The model under review builds one solid part; all positions refer to its coordinate system, in mm. Face numbers are marked on the shaded views. A direction names the side the tool comes from. Round coordinates to 2 decimals unless told otherwise and drop trailing zeros. Write each loop counter-clockwise with the first axis right and the second up, starting at its lowest first coordinate (ties: lowest second). Pieces come first, ordered by that corner, then holes. Notation, with made-up numbers: (65.5, -34) - (111.5, -34) arc R19 cw to (111.5, -27) - close; hole circle Ø8 at (-38, 10). An arc over 180 degrees is marked (long way). Return JSON: item names as keys, results as strings.
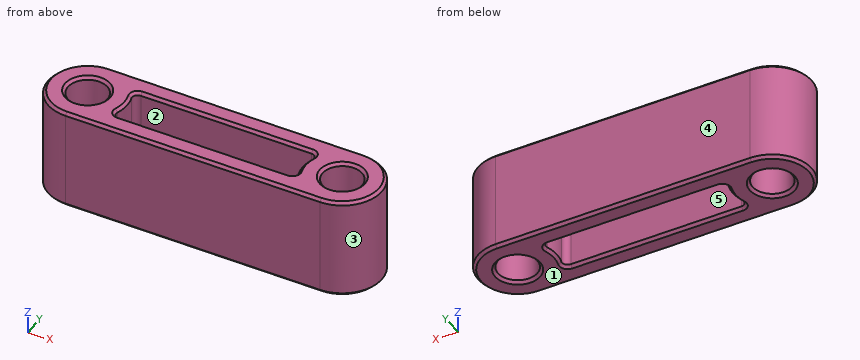
from build123d import *

# Parameters (mm, degrees)
SKETCH1_R           = 1.75
BOSS_EXTRUDE1_DEPTH = 9
FILLET1_R           = 0.5
CHAMFER2_SIZE       = 0.25


with BuildPart() as part:
    # Sketch1 → Boss-Extrude1 (new body)
    with BuildSketch(Plane.XY):
        with BuildLine():
            Line((-11.5, 3.5), (11.5, 3.5))
            ThreePointArc((11.5, 3.5), (15, 0), (11.5, -3.5))
            Line((11.5, -3.5), (-11.5, -3.5))
            ThreePointArc((-11.5, -3.5), (-15, 0), (-11.5, 3.5))
        make_face()
        with Locations((-11.5, 0)):
            Circle(SKETCH1_R, mode=Mode.SUBTRACT)
        with Locations((11.5, 0)):
            Circle(SKETCH1_R, mode=Mode.SUBTRACT)
        with BuildLine():
            Line((-8.468911087, 1.75), (8.468911087, 1.75))
            ThreePointArc((8.468911087, 1.75), (8, 0), (8.468911087, -1.75))
            Line((8.468911087, -1.75), (-8.468911087, -1.75))
            ThreePointArc((-8.468911087, -1.75), (-8, 0), (-8.468911087, 1.75))
        make_face(mode=Mode.SUBTRACT)
    extrude(amount=BOSS_EXTRUDE1_DEPTH)

    # Fillet1
    fillet1_edges = [part.edges().sort_by_distance(p)[0] for p in [
        (-8.468911087, 1.75, 4.5),
        (-8.468911087, -1.75, 4.5),
        (8.468911087, -1.75, 4.5),
        (8.468911087, 1.75, 4.5),
    ]]
    fillet(fillet1_edges, radius=FILLET1_R)

    # Chamfer2
    chamfer2_edges = [part.edges().sort_by_distance(p)[0] for p in [
        (9.75, 0, 0),
        (9.75, 0, 9),
        (15, 0, 9),
        (-13.25, 0, 0),
        (-13.25, 0, 9),
        (0, 3.5, 9),
        (0, -1.75, 0),
        (0, -1.75, 9),
        (8, 0, 0),
        (8, 0, 9),
        (0, 1.75, 0),
        (0, 1.75, 9),
        (-8, 0, 0),
        (-8, 0, 9),
        (8.105375255, -1.543150985, 0),
        (8.105375255, -1.543150985, 9),
        (8.105375255, 1.543150985, 0),
        (8.105375255, 1.543150985, 9),
        (-8.105375255, 1.543150985, 0),
        (-8.105375255, 1.543150985, 9),
        (-8.105375255, -1.543150985, 0),
        (-8.105375255, -1.543150985, 9),
        (-15, 0, 9),
        (0, 3.5, 0),
        (15, 0, 0),
        (0, -3.5, 0),
        (-15, 0, 0),
        (0, -3.5, 9),
    ]]
    chamfer(chamfer2_edges, length=CHAMFER2_SIZE)


solid = part.part
(1) Mouldability with a two-part tool opening along X and no side actions: class the marked faces 3, 4 and 5 as released by +X, released by -X, zero draft, split by the parting line, or undercut.
Filled in:
{"face 3": "released by +X", "face 4": "zero draft", "face 5": "undercut"}
(2) Add section B-B (y = 0). Give the number of separate pieces and of enclosed holes in the cut face, plus the area to 3 significant figures.
Filled in:
{"separate pieces": "4", "enclosed holes": "0", "area": "62.5 mm2"}
(3) Add section A-A (x = 3.5). Write out the cut boundary in (y, z).
Filled in:
{"outline": "(-3.5, 0.25) - (-3.25, 0) - (-2, 0) - (-1.75, 0.25) - (-1.75, 8.75) - (-2, 9) - (-3.25, 9) - (-3.5, 8.75) - close; (1.75, 0.25) - (2, 0) - (3.25, 0) - (3.5, 0.25) - (3.5, 8.75) - (3.25, 9) - (2, 9) - (1.75, 8.75) - close"}
(4) For the marked faces 1 and 2, list the 3-axis set-ups (+Z, -Z, +X, -X, +Y, -Y) from which the entire face can be reached by the end or side of a thin tool; tool diameter is ignored.
Filled in:
{"face 1": "-Z, +X, -X, +Y, -Y", "face 2": "+Z, -Z"}
(5) Add section C-C (z = 3). Write out the cut boundary in (x, y).
Filled in:
{"outline": "(-11.5, -3.5) - (11.5, -3.5) arc R3.5 ccw to (11.5, 3.5) - (-11.5, 3.5) arc R3.5 ccw to start; hole circle Ø3.5 at (-11.5, 0); hole (-8.18, -1.09) arc R0.5 ccw to (-7.7, -1.75) - (7.7, -1.75) arc R0.5 ccw to (8.18, -1.09) arc R3.5 cw to (8.18, 1.09) arc R0.5 ccw to (7.7, 1.75) - (-7.7, 1.75) arc R0.5 ccw to (-8.18, 1.09) arc R3.5 cw to start; hole circle Ø3.5 at (11.5, 0)"}
(6) Wall thickness on line 1 (Y direction, x = -11.5, z = 2); line 2 (X direction, y = 0.75, z = 4): over which ranges is each line inside the solid? List them lowest first.
Filled in:
{"line 1": "y = -3.5 to -1.75, 1.75 to 3.5", "line 2": "x = -14.92 to -13.08, -9.92 to -8.08, 8.08 to 9.92, 13.08 to 14.92"}
